```python
from build123d import *

# Parameters (mm, degrees)
SKETCH_2_R          = 1.5
EXTRUDE_1_DEPTH     = 3
EXTRUDE_START       = -3
EXTRUDE_2_DEPTH     = 3
FILLET_3_R          = 3
FILLET_4_R          = 10
FILLET_5_R          = 3
CUT_EXTRUDE_1_DEPTH = 9.5
FILLET_6_R          = 3
CUT_EXTRUDE_2_DEPTH = 256.693293577
CUT_EXTRUDE_3_DEPTH = 256.693293577
SKETCH_7_W          = 10
SKETCH_7_H          = 2
CUT_EXTRUDE_4_DEPTH = 256.693293577
FILLET_9_R          = 1
FILLET_10_R         = 3
SKETCH_8_R          = 6
EXTRUDE_3_DEPTH     = 3
SKETCH_9_R          = 3.5
CUT_EXTRUDE_5_DEPTH = 3
SKETCH_10_R         = 3.5
CUT_EXTRUDE_6_DEPTH = 3
EXTRUDE_6_DEPTH     = 3
EXTRUDE_7_DEPTH     = 3
EXTRUDE_8_DEPTH     = 3
FILLET_12_R         = 3
FILLET_13_R         = 20


with BuildPart() as part:
    # 草图2 → 凸台-拉伸1 (new body)
    # profile 1 of 3: a face of its own
    with BuildSketch(Plane(origin=(0, 0, 0), x_dir=(1, 0, 0), z_dir=(0, 1, 0))):
        with BuildLine():
            Line((-4, 27), (-4, 23))
            Line((-4, 23), (-4, 3))
            ThreePointArc((-4, 3), (0, 5), (4, 3))
            Line((4, 3), (4, 18.72063168))
            ThreePointArc((4, 18.72063168), (61.714912944, 58.202422296), (83.951238111, 124.5))
            Line((83.951238111, 124.5), (83.951238111, 241.5))
            Line((83.951238111, 241.5), (73.951238111, 241.5))
            Line((73.951238111, 241.5), (73.951238111, 124.5))
            ThreePointArc((73.951238111, 124.5), (52.067846257, 62.084766437), (-4, 27))
        make_face()
        with Locations(Location((0, 19, 0), (0, 0, 270))):
            Circle(SKETCH_2_R, mode=Mode.SUBTRACT)
    # profile 2 of 3: a face of its own
    with BuildSketch(Plane(origin=(0, 0, 0), x_dir=(1, 0, 0), z_dir=(0, 1, 0))):
        with BuildLine():
            ThreePointArc((4, 3), (0, 5), (-4, 3))
            Line((-4, 3), (-4, 0))
            Line((-4, 0), (-1.5, 0))
            ThreePointArc((-1.5, 0), (0, 1.5), (1.5, 0))
            Line((1.5, 0), (4, 0))
            Line((4, 0), (4, 3))
        make_face()
    # profile 3 of 3: a face of its own
    with BuildSketch(Plane(origin=(0, 0, 0), x_dir=(1, 0, 0), z_dir=(0, 1, 0))):
        with BuildLine():
            Line((-4, 0), (-4, 3))
            ThreePointArc((-4, 3), (-1.58113883, -4.74341649), (5, 0))
            ThreePointArc((5, 0), (4.74341649, 1.58113883), (4, 3))
            Line((4, 3), (4, 0))
            Line((4, 0), (1.5, 0))
            ThreePointArc((1.5, 0), (0, -1.5), (-1.5, 0))
            Line((-1.5, 0), (-4, 0))
        make_face()
    extrude(amount=EXTRUDE_1_DEPTH)

    # 草图3 → 凸台-拉伸2 (add)
    with BuildSketch(Plane(origin=(0, 3, 0), x_dir=(1, 0, 0), z_dir=(0, 1, 0)).offset(EXTRUDE_START)):
        with BuildLine():
            ThreePointArc((4, 3), (4.472135955, -2.236067977), (0, -5))
            Line((0, -5), (45, -5))
            Line((45, -5), (77.720510398, 88.012598271))
            ThreePointArc((77.720510398, 88.012598271), (68.645690453, 68.540478551), (55.957710685, 51.204649386))
            Line((55.957710685, 51.204649386), (39, 3))
            Line((39, 3), (4, 3))
        make_face()
    extrude(amount=EXTRUDE_2_DEPTH)

    # 圆角3
    fillet_3_edges = [part.edges().sort_by_distance(p)[0] for p in [
        (55.957710685, 1.5, -51.204649386),
    ]]
    fillet(fillet_3_edges, radius=FILLET_3_R)

    # 圆角4
    fillet_4_edges = [part.edges().sort_by_distance(p)[0] for p in [
        (39, 1.5, -3),
        (45, 1.5, 5),
    ]]
    fillet(fillet_4_edges, radius=FILLET_4_R)

    # 圆角5
    fillet_5_edges = [part.edges().sort_by_distance(p)[0] for p in [
        (4, 1.5, -3),
        (-4, 1.5, -3),
    ]]
    fillet(fillet_5_edges, radius=FILLET_5_R)

    # 草图4 → 切除-拉伸1 (cut)
    with BuildSketch(Plane(origin=(0, 3, 0), x_dir=(1, 0, 0), z_dir=(0, 1, 0))):
        with BuildLine():
            Line((40.866025404, -2), (44.299038106, 3.946152423))
            ThreePointArc((44.299038106, 3.946152423), (43.75, 5.995190528), (41.700961894, 5.446152423))
            Line((41.700961894, 5.446152423), (39.133974596, 1))
            Line((39.133974596, 1), (34, 1))
            ThreePointArc((34, 1), (32.5, -0.5), (34, -2))
            Line((34, -2), (40.866025404, -2))
        make_face()
    extrude(amount=-CUT_EXTRUDE_1_DEPTH, mode=Mode.SUBTRACT)

    # 圆角6
    fillet_6_edges = [part.edges().sort_by_distance(p)[0] for p in [
        (40.866025404, 1.5, 2),
        (39.133974596, 1.5, -1),
    ]]
    fillet(fillet_6_edges, radius=FILLET_6_R)

    # 草图5 → 切除-拉伸2 (cut, through all)
    with BuildSketch(Plane(origin=(0, 3, 0), x_dir=(1, 0, 0), z_dir=(0, 1, 0))):
        with BuildLine():
            Line((62.714846418, 67.264294142), (58.126234927, 60.711077788))
            ThreePointArc((58.126234927, 60.711077788), (56.037142206, 60.342714376), (55.668778794, 62.431807097))
            Line((55.668778794, 62.431807097), (60.257390285, 68.985023451))
            ThreePointArc((60.257390285, 68.985023451), (62.346483006, 69.353386863), (62.714846418, 67.264294142))
        make_face()
    extrude(amount=-CUT_EXTRUDE_2_DEPTH, mode=Mode.SUBTRACT)

    # 草图6 → 切除-拉伸3 (cut, through all)
    with BuildSketch(Plane(origin=(0, 3, 0), x_dir=(1, 0, 0), z_dir=(0, 1, 0))):
        with BuildLine():
            Line((78.951238111, 235.5), (78.951238111, 227.5))
            ThreePointArc((78.951238111, 227.5), (77.451238111, 226), (75.951238111, 227.5))
            Line((75.951238111, 227.5), (75.951238111, 235.5))
            ThreePointArc((75.951238111, 235.5), (77.451238111, 237), (78.951238111, 235.5))
        make_face()
        with BuildLine():
            Line((75.951238111, 165.5), (75.951238111, 157.5))
            ThreePointArc((75.951238111, 157.5), (77.451238111, 156), (78.951238111, 157.5))
            Line((78.951238111, 157.5), (78.951238111, 165.5))
            ThreePointArc((78.951238111, 165.5), (77.451238111, 167), (75.951238111, 165.5))
        make_face()
    extrude(amount=-CUT_EXTRUDE_3_DEPTH, mode=Mode.SUBTRACT)

    # 草图7 → 切除-拉伸4 (cut, through all)
    with BuildSketch(Plane(origin=(0, 3, 0), x_dir=(1, 0, 0), z_dir=(0, 1, 0))):
        with Locations((78.951238111, 240.5)):
            Rectangle(SKETCH_7_W, SKETCH_7_H)
    extrude(amount=-CUT_EXTRUDE_4_DEPTH, mode=Mode.SUBTRACT)

    # 圆角9
    fillet_9_edges = [part.edges().sort_by_distance(p)[0] for p in [
        (73.951238111, 1.5, -239.5),
    ]]
    fillet(fillet_9_edges, radius=FILLET_9_R)

    # 圆角10
    fillet_10_edges = [part.edges().sort_by_distance(p)[0] for p in [
        (83.951238111, 1.5, -239.5),
    ]]
    fillet(fillet_10_edges, radius=FILLET_10_R)

    # 草图8 → 凸台-拉伸3 (add)
    with BuildSketch(Plane(origin=(0, 3, 0), x_dir=(1, 0, 0), z_dir=(0, 1, 0))):
        Circle(SKETCH_8_R)
    extrude(amount=-EXTRUDE_3_DEPTH)

    # 草图9 → 切除-拉伸5 (cut)
    with BuildSketch(Plane(origin=(0, 3, 0), x_dir=(1, 0, 0), z_dir=(0, 1, 0))):
        with Locations(Location((0, 0, 0), (0, 0, 270))):
            Circle(SKETCH_9_R)
    extrude(amount=-CUT_EXTRUDE_5_DEPTH, mode=Mode.SUBTRACT)

    # 草图10 → 切除-拉伸6 (cut)
    with BuildSketch(Plane(origin=(0, 3, 0), x_dir=(1, 0, 0), z_dir=(0, 1, 0))):
        with Locations(Location((0, 19, 0), (0, 0, 270))):
            Circle(SKETCH_10_R)
    extrude(amount=-CUT_EXTRUDE_6_DEPTH, mode=Mode.SUBTRACT)

    # 草图12 → 凸台-拉伸6 (add)
    with BuildSketch(Plane(origin=(0, 3, 0), x_dir=(1, 0, 0), z_dir=(0, 1, 0))):
        Polygon((4, 6), (4, 18.72063168), (7.464101615, 20.72063168), align=None)
    extrude(amount=-EXTRUDE_6_DEPTH)

    # 草图14 → 凸台-拉伸7 (add)
    with BuildSketch(Plane(origin=(0, 3, 0), x_dir=(1, 0, 0), z_dir=(0, 1, 0))):
        Polygon((-4, 27), (-6, 0), (-4, 4.472135955), align=None)
    extrude(amount=-EXTRUDE_7_DEPTH)

    # 草图15 → 凸台-拉伸8 (add)
    with BuildSketch(Plane(origin=(0, 3, 0), x_dir=(1, 0, 0), z_dir=(0, 1, 0))):
        with BuildLine():
            Line((-5.135061392, 11.676671214), (-4, 27))
            ThreePointArc((-4, 27), (-8.919833963, 19.660728442), (-5.135061392, 11.676671214))
        make_face()
    extrude(amount=-EXTRUDE_8_DEPTH)

    # 圆角12
    fillet_12_edges = [part.edges().sort_by_distance(p)[0] for p in [
        (-4, 1.5, -27),
        (-5.135061392, 1.5, -11.676671214),
    ]]
    fillet(fillet_12_edges, radius=FILLET_12_R)

    # 圆角13
    fillet_13_edges = [part.edges().sort_by_distance(p)[0] for p in [
        (7.221005183, 1.5, -19.687598172),
    ]]
    fillet(fillet_13_edges, radius=FILLET_13_R)


solid = part.part
```
Design review of the part built by this model. Coordinates are the model's own, in mm. A direction names the side the tool comes from. Coordinates: 2 decimals unless noted, no trailing zeros. Order: outer loops, then holes, each group sorted by start corner. A loop starts at its lowest first (then second) coordinate and runs counter-clockwise, first axis right, second up. Notation, with made-up numbers: M 36.5,-12 L 65.5,-12 A6 cw 65.5,-8 Z; hole C 3.5,33.5 d11. An arc over 180 degrees is marked long. Answer as a JSON object with one key per item and string values. Group by question number.
1) Add section B-B, the plane x = 27. Write out the cut boundary in (y, z).
2) Wall thickness on L1, parallel to X at y = 2, z = -19; L2, parallel to X at y = 2, z = 0; L3, parallel to Z at x = 24, y = 1.15: over which ranges is each line inside the solid? List them lowest first.
3) Mouldability with a two-part tool opening along Z and no side actions: class faces 3 (the cylindrical face through (82.34, 1.48, -105.74)), 4 (the cylindrical face through (8.88, 1.48, -17.47)), 5 (the cylindrical face through (-8.863, 1.521, -20.2)), 6 (the cylindrical face through (-1.341, 1.521, -15.767)) as pulls with the +Z half, pulls with the -Z half, needs draft (parallel to the pull), parting line crosses it, or undercut.
4) Add section C-C, the plane z = -18. Write out the cut boundary in (x, y).
5) Add section D-D, the plane y = 2.05. Count the separate pieces of the cut face and the enclosed holes in it, then the cut area to 3 significant figures.
6) Tool access review of faces 1 (the flat face through (68, 0, -81)), 2 (the flat face through (57.93, 1.52, -65.66)): name each direction out of +Z, -Z, +X, -X, +Y, -Y from which nothing blocks a thin tool from reaching the whole face with its end or side.
7) Add section A-A, the plane x = 0. Write out the cut boundary in (y, z).
8) For pin 1 (1.5 mm diameter, centred on x = 37.5, y = 1, fed in from -Z); pin 2 (1.5 mm diameter, centred on y = 2, z = -161.5, fed in from -X); pin 3 (1.5 mm diameter, centred on x = 16, y = 1.5, fed in from -Z); pin 4 (10 mm diameter, centred on x = 70, z = -86.5, fed in from -Y), all flat-tipped, find the tip position at first contact; note any pin that passes through.
Computed values:
{
 "1": {"outline": "M 0,-39.76 L 3,-39.76 L 3,-28.17 L 0,-28.17 Z; M 0,-3 L 3,-3 L 3,5 L 0,5 Z"},
 "2": {"L1": "x = -8.94 to -3.5, 3.5 to 10.3, 44.63 to 53.44", "L2": "x = -6 to -3.5, 3.5 to 32.59, 42.02 to 46.58", "L3": "z = -37.95 to -26.58, -3 to 5"},
 "3": {"face 3": "pulls with the +Z half", "face 4": "undercut", "face 5": "parting line crosses it", "face 6": "undercut"},
 "4": {"outline": "M -8.89,0 L -3.35,0 L -3.35,3 L -8.89,3 Z; M 3.35,0 L 9.34,0 L 9.34,3 L 3.35,3 Z; M 44.28,0 L 53.09,0 L 53.09,3 L 44.28,3 Z"},
 "5": {"separate pieces": "1", "enclosed holes": "7", "area": "3,560 mm^2"},
 "6": {"face 1": "+Z, -Z, +X, -X, -Y", "face 2": "+Y, -Y"},
 "7": {"outline": "M 0,-27.99 L 3,-27.99 L 3,-22.5 L 0,-22.5 Z; M 0,-15.5 L 3,-15.5 L 3,-3.5 L 0,-3.5 Z; M 0,3.5 L 3,3.5 L 3,6 L 0,6 Z"},
 "8": {"pin 1": "stops at z = -47.94", "pin 2": "stops at x = 73.95", "pin 3": "stops at z = -34.15", "pin 4": "stops at y = 0"}
}
